Read the model definition and answer for the solid it produces. Units are mm, in the model's axes. Face numbers are marked on the shaded views. Round coordinates to 2 decimals unless told otherwise and drop trailing zeros. Order: outer loops, then holes, each group sorted by start corner. A loop starts at its lowest first (then second) coordinate and runs counter-clockwise, first axis right, second up. Notation, with made-up numbers: (-35.75, -19.75) - (-14.75, -19.75) arc R13 ccw to (-14.75, -13.75) - close; hole circle Ø4 at (66.25, 63). An arc over 180 degrees is marked (long way). One line per question, with ' | ' between items. Start each with the question number.
1) Straight lines are drawn through the part: line 1 (Y direction, x = 30, z = -0.3); line 2 (Z direction, x = 2, y = 338); line 3 (Z direction, x = 34, y = 331). For each, find the intervals that lie inside material, in ascending order. Write a range as from..to.
2) The part is cut by section C-C, the plane x = 60. Count the separate pieces of the cut face and the enclosed holes in it, plus the area to 3 significant figures.
3) The mould has two halves that part along Z. Classify the marked faces 1, 2, 3 and 4: pulls with the +Z half, pulls with the -Z half, needs draft (parallel to the pull), parting line crosses it, or undercut.
4) Flat-ended cylindrical pins translate along their axes: pin 1 (6 mm diameter, centred on y = 338, z = -102, fed in from -X); pin 2 (5 mm diameter, centred on y = 349, z = -96, fed in from -X); pin 3 (10 mm diameter, centred on y = 304, z = -57, fed in from -X); pin 4 (12 mm diameter, centred on x = 5, y = 311, fed in from -Z). Find the tip coordinate at first contact, or state that the pin passes through.
5) The part is cut by section B-B, the plane z = -86.5. Give the vertices of the cut face in (x, y).
6) The part is cut by section A-A, the plane y = 362.5. Give the vertices of the cut face in (x, z).
from build123d import *

# Parameters (mm, degrees)
EXTRUDE_1_DEPTH     = 108
SKETCH_2_R          = 27
EXTRUDE_2_DEPTH     = 18
EXTRUDE_3_DEPTH     = 6
SKETCH_4_R          = 24.5
EXTRUDE_4_DEPTH     = 2
SKETCH_5_R          = 23.5
EXTRUDE_5_DEPTH     = 4
SKETCH_7_R          = 1.6
SKETCH_7_R_2        = 1.45
SKETCH_7_R_3        = 1.464509856
CUT_EXTRUDE_1_DEPTH = 14
SKETCH_8_R          = 14.5
CUT_EXTRUDE_2_DEPTH = 1


with BuildPart() as part:
    # 스케치1 → 보스-돌출1 (new body)
    with BuildSketch(Plane.XY):
        Polygon((-6.769552622, 334.414213562), (-6.769552622, 331.585786438), (28.585786438, 296.230447378), (31.414213562, 296.230447378), (66.769552622, 331.585786438), (66.769552622, 334.414213562), (31.414213562, 369.769552622), (28.585786438, 369.769552622), align=None)
    extrude(amount=-EXTRUDE_1_DEPTH)

    # 스케치2 → 보스-돌출2 (add)
    with BuildSketch(Plane(origin=(0, 0, -108), x_dir=(-1, 0, 0), z_dir=(0, 0, -1))):
        with Locations(Location((-30, 333, 0), (0, 0, 135))):
            Circle(SKETCH_2_R)
    extrude(amount=EXTRUDE_2_DEPTH)

    # 스케치3 → 보스-돌출3 (add)
    with BuildSketch(Plane(origin=(0, 0, -126), x_dir=(-1, 0, 0), z_dir=(0, 0, -1))):
        Polygon((6.769552622, 331.585786438), (6.769552622, 334.414213562), (-28.585786438, 369.769552622), (-31.414213562, 369.769552622), (-66.769552622, 334.414213562), (-66.769552622, 331.585786438), (-31.414213562, 296.230447378), (-28.585786438, 296.230447378), align=None)
    extrude(amount=EXTRUDE_3_DEPTH)

    # 스케치4 → 보스-돌출4 (add)
    with BuildSketch(Plane(origin=(0, 0, -132), x_dir=(-1, 0, 0), z_dir=(0, 0, -1))):
        with Locations((-30, 333)):
            Circle(SKETCH_4_R)
    extrude(amount=EXTRUDE_4_DEPTH)

    # 스케치5 → 보스-돌출5 (add)
    with BuildSketch(Plane(origin=(0, 0, -134), x_dir=(-1, 0, 0), z_dir=(0, 0, -1))):
        with Locations((-30, 333)):
            Circle(SKETCH_5_R)
    extrude(amount=EXTRUDE_5_DEPTH)

    # 스케치7 → 컷-돌출1 (cut)
    with BuildSketch(Plane(origin=(-132.408116908, 132.408116908, 0), x_dir=(0, 0, -1), z_dir=(0.7071067811863883, -0.7071067811867069, 0))):
        with Locations(Location((105, 274.679761571, 0), (0, 0, 90))):
            Circle(SKETCH_7_R)
        with Locations(Location((93, 274.679761571, 0), (0, 0, 90))):
            Circle(SKETCH_7_R_2)
        with Locations(Location((81, 274.679761571, 0), (0, 0, 90))):
            Circle(SKETCH_7_R_2)
        with Locations(Location((69, 274.679761571, 0), (0, 0, 90))):
            Circle(SKETCH_7_R_2)
        with Locations(Location((57, 274.679761571, 0), (0, 0, 90))):
            Circle(SKETCH_7_R_2)
        with Locations(Location((45, 274.679761571, 0), (0, 0, 90))):
            Circle(SKETCH_7_R_2)
        with Locations(Location((33, 274.679761571, 0), (0, 0, 90))):
            Circle(SKETCH_7_R_2)
        with Locations(Location((21, 274.679761571, 0), (0, 0, 90))):
            Circle(SKETCH_7_R_3)
        with Locations(Location((21, 238.679761571, 0), (0, 0, 90))):
            Circle(SKETCH_7_R_2)
        with Locations(Location((33, 238.679761571, 0), (0, 0, 90))):
            Circle(SKETCH_7_R_2)
        with Locations(Location((45, 238.679761571, 0), (0, 0, 90))):
            Circle(SKETCH_7_R_2)
        with Locations(Location((57, 238.679761571, 0), (0, 0, 90))):
            Circle(SKETCH_7_R_2)
        with Locations(Location((69, 238.679761571, 0), (0, 0, 90))):
            Circle(SKETCH_7_R_2)
        with Locations(Location((81, 238.679761571, 0), (0, 0, 90))):
            Circle(SKETCH_7_R_2)
        with Locations(Location((93, 238.679761571, 0), (0, 0, 90))):
            Circle(SKETCH_7_R_2)
        with Locations(Location((105, 238.679761571, 0), (0, 0, 90))):
            Circle(SKETCH_7_R)
    extrude(amount=-CUT_EXTRUDE_1_DEPTH, mode=Mode.SUBTRACT)

    # 스케치8 → 컷-돌출2 (cut)
    with BuildSketch(Plane.XY):
        with Locations((30, 333)):
            Circle(SKETCH_8_R)
    extrude(amount=-CUT_EXTRUDE_2_DEPTH, mode=Mode.SUBTRACT)


solid = part.part
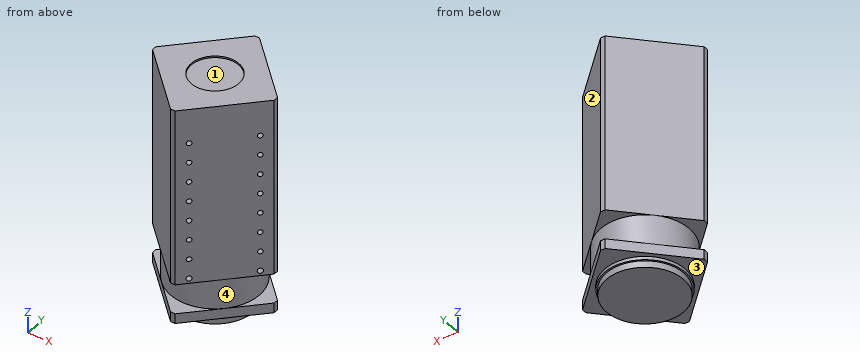
Values:
1) line 1: y = 296.23..318.5, 347.5..369.77 | line 2: z = -132..-126, -108..0 | line 3: z = -138..-1
2) separate pieces: 2 | enclosed holes: 8 | area: 1,790 mm^2
3) face 1: pulls with the +Z half | face 2: needs draft | face 3: pulls with the -Z half | face 4: undercut
4) pin 1: stops at x = -6.18 | pin 2: stops at x = 5.32 | pin 3: stops at x = 15.82 | pin 4: passes through
5) outline: (-6.77, 331.59) - (28.59, 296.23) - (31.41, 296.23) - (66.77, 331.59) - (66.77, 334.41) - (31.41, 369.77) - (28.59, 369.77) - (-6.77, 334.41) - close
6) outline: (21.32, -132) - (38.68, -132) - (38.68, -126) - (21.32, -126) - close; (21.32, -108) - (38.68, -108) - (38.68, 0) - (21.32, 0) - close
